Autodesk Inventor part; units mm, degrees
ref_plane "YZ Plane" through (0, 0, 0) normal (1, 0, 0) x (0, 1, 0)
ref_plane "XZ Plane" through (0, 0, 0) normal (0, 1, 0) x (-1, 0, 0)
ref_plane "XY Plane" through (0, 0, 0) normal (0, 0, 1) x (1, 0, 0)
sketch "Sketch1" plane through (0, 0, 0) normal (0, 0, 1) x (1, 0, 0)
  line L0 (25.4, 25.4) -> (-25.4, 25.4)
  line L1 (-25.4, 25.4) -> (-25.4, -25.4)
  line L2 (-25.4, -25.4) -> (25.4, -25.4)
  line L3 (25.4, -25.4) -> (25.4, 25.4)
  line L4 (25.4, 25.4) -> (-25.4, -25.4) construction
  line L5 (-25.4, 25.4) -> (25.4, -25.4) construction
  point P0 (0, 0)
  dimension "d0" = 50.8
  dimension "d1" = 50.8
extrude "Plate1" add sketch "Sketch1" along normal blind 3.048
sketch "Sketch2" plane through (-28.448, -25.4, 6.096) normal (-1, 0, 0) x (0, -1, 0)
  line L0 (-50.8, 0) -> (0, 0)
  line L1 (0, 0) -> (0, 50.8)
  line L2 (0, 50.8) -> (-50.8, 50.8)
  line L3 (-50.8, 50.8) -> (-50.8, 0)
edge flange "Flange1" height 56.896 angle 90 thickness 3.048 bend radius 3.048 thickness toward (-1, 0, 0) relief tear relief width 3.048 relief depth 1.524 edges at (-25.4, 0, 3.048) wall of the first edge with corners at (-28.448, 25.4, 6.096) (-28.448, -25.4, 6.096) (-28.448, -25.4, 56.896) (-28.448, 25.4, 56.896)
bend "Bend1"
corner "Corner1"
sketch "Sketch3" plane through (-28.448, -25.4, 56.896) normal (1, 0, 0) x (0, 0, -1)
  line L0 (50.8, 0) -> (50.8, 50.8) construction
  line L1 (0, 50.8) -> (50.8, 50.8) construction
  line L2 (0, 50.8) -> (0, 0) construction
  line L3 (0, 0) -> (50.8, 0) construction
  point P0 (56.896, 25.4)
  point P1 (38.1, 38.1)
  point P2 (38.1, 12.7)
  point P3 (12.7, 38.1)
  point P4 (12.7, 12.7)
  dimension "d13" = 12.7
  dimension "d14" = 12.7
  dimension "d17" = 25.4
  dimension "d20" = 25.4
hole "Hole1" at (-28.448, 12.7, 18.796) at (-28.448, -12.7, 18.796) at (-28.448, 12.7, 44.196) at (-28.448, -12.7, 44.196) direction (-1, 0, 0) diameter 5.1054 end through all
sketch "Sketch4" plane through (0, 0, 3.048) normal (0, 0, 1) x (1, 0, 0)
  line L0 (-25.4, 25.4) -> (25.4, 25.4) construction
  line L1 (-25.4, -25.4) -> (-25.4, 25.4) construction
  line L2 (25.4, -25.4) -> (-25.4, -25.4) construction
  line L3 (25.4, 25.4) -> (25.4, -25.4) construction
  point P0 (0, 0)
  point P1 (-12.7, 12.7)
  point P2 (12.7, 12.7)
  point P3 (-12.7, -12.7)
  point P4 (12.7, -12.7)
  dimension "d30" = 12.7
  dimension "d31" = 12.7
  dimension "d34" = 25.4
  dimension "d37" = 25.4
hole "Hole2" at (-12.7, 12.7, 3.048) at (12.7, 12.7, 3.048) at (-12.7, -12.7, 3.048) at (12.7, -12.7, 3.048) direction (0, 0, -1) diameter 5.1054 end through all
equation "\"d28\" = Thickness"
equation "\"d2\" = Thickness"
equation "\"d3\" = BendReliefWidth"
equation "\"d4\" = BendReliefDepth"
equation "\"d5\" = MinimumRemnant"
equation "\"d6\" = TransitionRadius"
equation "\"d9\" = BendRadius"
equation "\"d10\" = CornerReliefSize"
equation "\"d11\" = GapSize"
equation "\"d12\" = JacobiRadiusSize"
equation "\"BendRadius\" = Thickness"
equation "\"BendReliefWidth\" = Thickness"
equation "\"BendReliefDepth\" = 0.5 * Thickness"
equation "\"CornerReliefSize\" = 4 * Thickness"
equation "\"MinimumRemnant\" = 2 * Thickness"
equation "\"TransitionRadius\" = BendRadius"
equation "\"JacobiRadiusSize\" = BendRadius"
equation "\"GapSize\" = Thickness"
properties part number "hopper_side_barcket"
The model under review builds one solid part; all positions refer to its coordinate system, in mm. A direction names the side the tool comes from. Give positions to 0.01 mm unless a question says otherwise; leave off trailing zeros. Write each loop counter-clockwise with the first axis right and the second up, starting at its lowest first coordinate (ties: lowest second). Pieces come first, ordered by that corner, then holes. Notation, with made-up numbers: (43, 10) -> (102, 10) arc R22 ccw to (102, 39) -> close; hole circle Ø4 at (-34, 86). An arc over 180 degrees is marked (long way). Answer in a Markdown table with one row per item.
1) Clearance check with flat-ended pins moving along their axes: P1, Ø8, axis at y = 11, z = 29, coming from the +X side; P2, Ø10, axis at x = -10.5, y = -1, coming from the +Z side. State where each tip first meets the part, or that it passes through.
Worked answers:
| item | result |
|---|---|
| P1 | x = -28.45 |
| P2 | z = 3.05 |
2) Tool access review of faces 1 (the flat face through (-28.448, 0, 31)), 2 (the cylindrical face through (-29.993, 12.588, 46.746)): name each direction out of +Z, -Z, +X, -X, +Y, -Y from which nothing blocks a thin tool from reaching the whole face with its end or side.
Worked answers:
| item | result |
|---|---|
| face 1 | +Z, +X, +Y, -Y |
| face 2 | +X, -X |
3) For L1, parallel to Y at x = 12.7, z = 1.05; L2, parallel to Z at x = -30, y = 12; L3, parallel to X at y = 12.7, z = 0.85, list the stretches that pass through material, from the lowest coordinate up. Write a range as [from, to].
Worked answers:
| item | result |
|---|---|
| L1 | [-25.4, -15.25], [-10.15, 10.15], [15.25, 25.4] |
| L2 | [2.1, 16.34], [21.25, 41.74], [46.65, 56.9] |
| L3 | [-28.5, -15.25], [-10.15, 10.15], [15.25, 25.4] |
4) Add section A-A on y = 12.7. State the section outline as (x, z) points, plus the area to 3 significant figures.
Worked answers:
| item | result |
|---|---|
| outline | (-31.5, 6.1) arc R6.1 ccw to (-25.4, 0) -> (-15.25, 0) -> (-15.25, 3.05) -> (-25.4, 3.05) arc R3.05 cw to (-28.45, 6.1) -> (-28.45, 16.24) -> (-31.5, 16.24) -> close; (-31.5, 21.35) -> (-28.45, 21.35) -> (-28.45, 41.64) -> (-31.5, 41.64) -> close; (-31.5, 46.75) -> (-28.45, 46.75) -> (-28.45, 56.9) -> (-31.5, 56.9) -> close; (-10.15, 0) -> (10.15, 0) -> (10.15, 3.05) -> (-10.15, 3.05) -> close; (15.25, 0) -> (25.4, 0) -> (25.4, 3.05) -> (15.25, 3.05) -> close |
| area | 269 mm² |
5) Add section C-C on z = 19. State the section outline as (x, y) points, plus the area to 3 significant figures.
Worked answers:
| item | result |
|---|---|
| outline | (-31.5, -25.4) -> (-28.45, -25.4) -> (-28.45, -15.24) -> (-31.5, -15.24) -> close; (-31.5, -10.16) -> (-28.45, -10.16) -> (-28.45, 10.16) -> (-31.5, 10.16) -> close; (-31.5, 15.24) -> (-28.45, 15.24) -> (-28.45, 25.4) -> (-31.5, 25.4) -> close |
| area | 124 mm² |
6) Add section B-B on x = -12.7. State the section outline as (y, z) points, plus the area to 3 significant figures.
Worked answers:
| item | result |
|---|---|
| outline | (-25.4, 0) -> (-15.25, 0) -> (-15.25, 3.05) -> (-25.4, 3.05) -> close; (-10.15, 0) -> (10.15, 0) -> (10.15, 3.05) -> (-10.15, 3.05) -> close; (15.25, 0) -> (25.4, 0) -> (25.4, 3.05) -> (15.25, 3.05) -> close |
| area | 124 mm² |
7) Mouldability with a two-part tool opening along X and no side actions: class faces 3 (the cylindrical face through (13.678, 10.342, 1.503)), 4 (the flat face through (0, 0, 3.048)), 5 (the cylindrical face through (-29.758, -0.356, 1.833)) as +X half, -X half, draft (parallel to the pull), parting line (faces both ways), or undercut.
Worked answers:
| item | result |
|---|---|
| face 3 | undercut |
| face 4 | draft |
| face 5 | -X half |
8) Add section D-D on y = -20.5. State the section outline as (x, z) points.
Worked answers:
| item | result |
|---|---|
| outline | (-31.5, 6.1) arc R6.1 ccw to (-25.4, 0) -> (25.4, 0) -> (25.4, 3.05) -> (-25.4, 3.05) arc R3.05 cw to (-28.45, 6.1) -> (-28.45, 56.9) -> (-31.5, 56.9) -> close |
